Part model, mm, in its own coordinate system. Coordinates: 2 decimals unless noted, no trailing zeros. Loops run counter-clockwise (first coordinate to the right, second up) from the corner with the lowest first, then second, coordinate; pieces in that order, holes last. Notation, with made-up numbers: M -30.75,51.25 L -5.75,51.25 A24 cw -5.75,74.25 Z; hole C 68.5,42.5 d9. An arc over 180 degrees is marked long. Use a Markdown table: item, result. Add a question column.
1) Band-saw the part on C-C (x = 114.5). List the corners of the cut face in (y, z).
2) Band-saw the part on B-B (y = 246). List the corners of the cut face in (x, z).
3) Wall check: probe 1 along X at (y, z) = (218, 7); probe 2 along Y at (x, z) = (140.5, 24); probe 3 along Z at (x, y) = (-28, 297). Give the ranges that are in metal, low to high. Write a range as from..to.
4) Pin check, flat tips, straight feed: pin 1 Ø14.5 at (x, y) = (175, 283) entering from +Z; pin 2 Ø4 at (x, z) = (-100, 15) entering from +Y; pin 3 Ø1.5 at (x, z) = (-7.5, 15) entering from +Y. Stop position of each tip, or through.
5) Band-saw the part on A-A (x = -66.5). List the corners of the cut face in (y, z), plus the area to 3 significant figures.
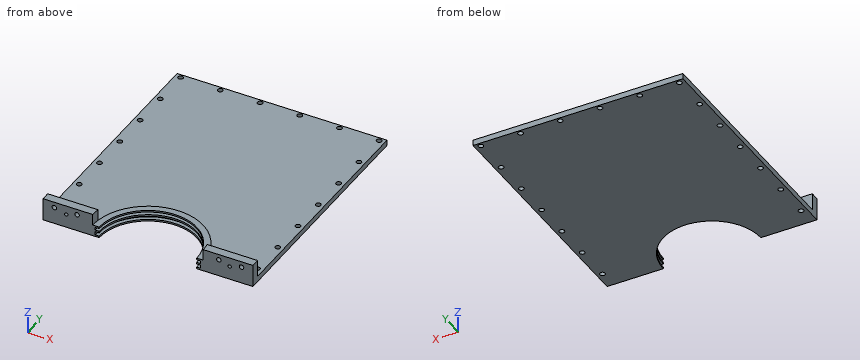
Autodesk Inventor part; units mm, degrees
ref_plane "РабПлоскость1" through (0, 0, 0) normal (0, 0, 1) x (1, 0, 0)
ref_plane "YZ Plane" through (0, 0, 0) normal (1, 0, 0) x (0, 1, 0)
ref_plane "XZ Plane" through (0, 0, 0) normal (0, 1, 0) x (-1, 0, 0)
ref_plane "РабПлоскость1" through (0, 0, 0) normal (0, 0, 1) x (1, 0, 0)
sketch "Эскиз1" plane through (0, 0, 0) normal (0, 0, 1) x (1, 0, 0)
  line L0 (185, -75) -> (185, 325)
  line L1 (165, 340) -> (165, -75)
  arc A0 (-165, -75) -> (165, -75) centre (0, -75) ccw
  line L2 (-165, -75) -> (-165, 340)
  line L3 (-185, 325) -> (-185, -75)
  arc A1 (-185, -75) -> (185, -75) centre (0, -75) ccw
  line L4 (185, -75) -> (97.5, -75)
  line L5 (-97.5, -75) -> (-185, -75)
  line L6 (-185, -75) -> (185, -75)
  line L7 (-185, 340) -> (-185, 355)
  line L8 (-185, 355) -> (185, 355)
  line L9 (185, 355) -> (185, 338)
  line L10 (185, 325) -> (230, 325)
  line L11 (230, 325) -> (230, 340)
  line L12 (230, 340) -> (165, 340)
  line L13 (-165, 340) -> (-230, 340)
  line L14 (-230, 340) -> (-230, 325)
  line L15 (-230, 325) -> (-185, 325)
  line L16 (-185, 340) -> (-185, 325)
  line L17 (185, 340) -> (185, 325)
  point P0 (0, 0)
  point P1 (-97.5, -75)
  point P2 (165, -75)
  point P3 (-165, -75)
  point P4 (-185, -75)
  point P5 (-165, -75)
  point P6 (185, -75)
  dimension "d0" = 15
  dimension "d1" = 370
extrude "Выдавливание1" add sketch "Эскиз1" along normal blind 10 contours L4 L1 L12 L9 L17 L0 | L3 L16 L13 L2 L5 | L4 L6 L5 L2 L13 L7 L8 L9 L12 L1
sketch "Эскиз2" plane through (0, 0, 10) normal (0, 0, 1) x (1, 0, 0)
  arc A0 (-96.3392, -90) -> (96.3392, -90) centre (0, -75) ccw
  arc A1 (-86, -75) -> (86, -75) centre (0, -75) ccw
  circle A2 centre (0, -75) radius 86
  line L0 (-185, -75) -> (185, -75)
  line L1 (-97.3373, -75) -> (97.3373, -75)
  circle A3 centre (0, -75) radius 97.3373
  point P0 (0, 0)
  point P1 (86, -75)
  point P2 (-165, -75)
  point P3 (165, -75)
extrude "Выдавливание2" add sketch "Эскиз2" along normal blind 10 contours L0 A3 A2
sketch "Эскиз3" plane through (0, 0, 10) normal (0, 0, 1) x (1, 0, 0)
  arc A0 (86, -75) -> (-86, -75) centre (0, -75) ccw
  line L0 (185, 355) -> (-185, 355)
  line L1 (-185, 355) -> (-185, -75)
  arc A1 (97.3373, -75) -> (-97.3373, -75) centre (0, -75) ccw
  line L2 (-86, -75) -> (86, -75)
  line L3 (97.3373, -75) -> (185, -75)
  line L4 (185, -75) -> (185, 355)
  line L5 (-185, -75) -> (-97.3373, -75)
  point P0 (0, 0)
extrude "Выдавливание3" cut sketch "Эскиз3" against normal through all contours L2 A0
sketch "Эскиз8" plane through (0, 0, 10) normal (0, 0, 1) x (1, 0, 0)
  line L0 (-185, 355) -> (-185, -75)
  line L1 (-185, 355) -> (-175, 355)
  line L2 (185, 355) -> (-185, 355)
  line L3 (-175, 355) -> (-175, 348)
  point P0 (0, 0)
hole "Отверстие1" at (-175, 348, 10) direction (0, 0, -1) diameter 9 end through all
pattern_linear "Прямоуг.массив1" count 7 spacing 65 along (0, -1, 0) of "Отверстие1"
mirror "Зеркальное отражение1" about plane through (0, 0, 0) normal (1, 0, 0) of "Отверстие1", "Прямоуг.массив1"
pattern_linear "Прямоуг.массив2" count 5 spacing 70 along (1, 0, 0) of "Отверстие1"
sketch "Эскиз9" plane through (0, 0, 10) normal (0, 0, 1) x (1, 0, 0)
  circle A0 centre (105, 348) radius 4.5
  circle A1 centre (35, 348) radius 4.5
  circle A2 centre (-35, 348) radius 4.5
  circle A3 centre (-105, 348) radius 4.5
  circle A4 centre (175, -42) radius 4.5
  circle A5 centre (175, 23) radius 4.5
  circle A6 centre (175, 88) radius 4.5
  circle A7 centre (175, 153) radius 4.5
  circle A8 centre (175, 218) radius 4.5
  circle A9 centre (175, 283) radius 4.5
  circle A10 centre (175, 348) radius 4.5
  circle A11 centre (-175, -42) radius 4.5
  circle A12 centre (-175, 23) radius 4.5
  circle A13 centre (-175, 88) radius 4.5
  circle A14 centre (-175, 153) radius 4.5
  circle A15 centre (-175, 218) radius 4.5
  circle A16 centre (-175, 283) radius 4.5
  circle A17 centre (-175, 348) radius 4.5
  arc A18 (97.3373, -75) -> (-97.3373, -75) centre (0, -75) ccw
  line L0 (97.3373, -75) -> (185, -75)
  line L1 (185, -75) -> (185, 355)
  line L2 (185, 355) -> (-185, 355)
  line L3 (-185, 355) -> (-185, -75)
  line L4 (-185, -75) -> (-97.3373, -75)
  line L5 (-185, -75) -> (-185, -60)
  line L6 (-185, 355) -> (-185, -75)
  line L7 (-185, -60) -> (-96.1746, -60)
  arc A19 (97.3373, -75) -> (-97.3373, -75) centre (0, -75) ccw
  line L8 (185, -75) -> (185, 355)
  line L9 (185, -75) -> (185, -60)
  line L10 (185, -60) -> (96.1746, -60)
  point P0 (0, 0)
  point P1 (-96.1746, -60)
  dimension "d31" = 15
  dimension "d32" = 15
extrude "Выдавливание7" add sketch "Эскиз9" along normal blind 30 contours A18 L10 L1 L0 | A18 L4 L3 L7
sketch "Эскиз10" plane through (-185, -60, 10) normal (0, 1, 0) x (1, 0, 0)
  circle A0 centre (20, -20) radius 4
  circle A1 centre (41, -14) radius 3
  circle A2 centre (60, -20) radius 4
  circle A3 centre (310, -20) radius 4
  circle A4 centre (329, -14) radius 3
  circle A5 centre (350, -20) radius 4
  point P0 (185, 10)
extrude "Выдавливание8" cut sketch "Эскиз10" against normal blind 30
sketch "Эскиз11" plane through (86, -75, 0) normal (0, -1, 0) x (1, 0, 0)
  line L0 (7, 17) -> (0, 17)
  line L1 (7, 12) -> (7, 17)
  line L2 (0, 12) -> (7, 12)
  line L3 (7, 9) -> (0, 9)
  line L4 (7, 3) -> (7, 9)
  line L5 (0, 3) -> (7, 3)
  line L6 (-86, 0) -> (-86, 42)
  line L7 (0, 17) -> (0, 3)
revolve "Вращение2" cut sketch "Эскиз11" angle 360 about axis through (0, -75, 0) along (0, 0, 1)
properties part number "Крышка стенки картера верх" material "Чугун, серый"
Entries:
| question | item | result |
|---|---|---|
| 1 | outline | M -75,0 L 355,0 L 355,10 L -60,10 L -60,40 L -75,40 Z |
| 2 | outline | M -185,0 L 185,0 L 185,10 L -185,10 Z |
| 3 | probe 1 | -185..-179.5, -170.5..170.5, 179.5..185 |
| 3 | probe 2 | -75..-60 |
| 3 | probe 3 | 0..10 |
| 4 | pin 1 | z = 10 |
| 4 | pin 2 | y = -60 |
| 4 | pin 3 | y = 22.1 |
| 5 | outline | M -20.47,0 L 355,0 L 355,10 L -3.92,10 L -3.92,20 L -20.47,20 L -20.47,17 L -9.99,17 L -9.99,12 L -20.47,12 L -20.47,9 L -9.99,9 L -9.99,3 L -20.47,3 Z |
| 5 | area | 3,800 mm2 |
